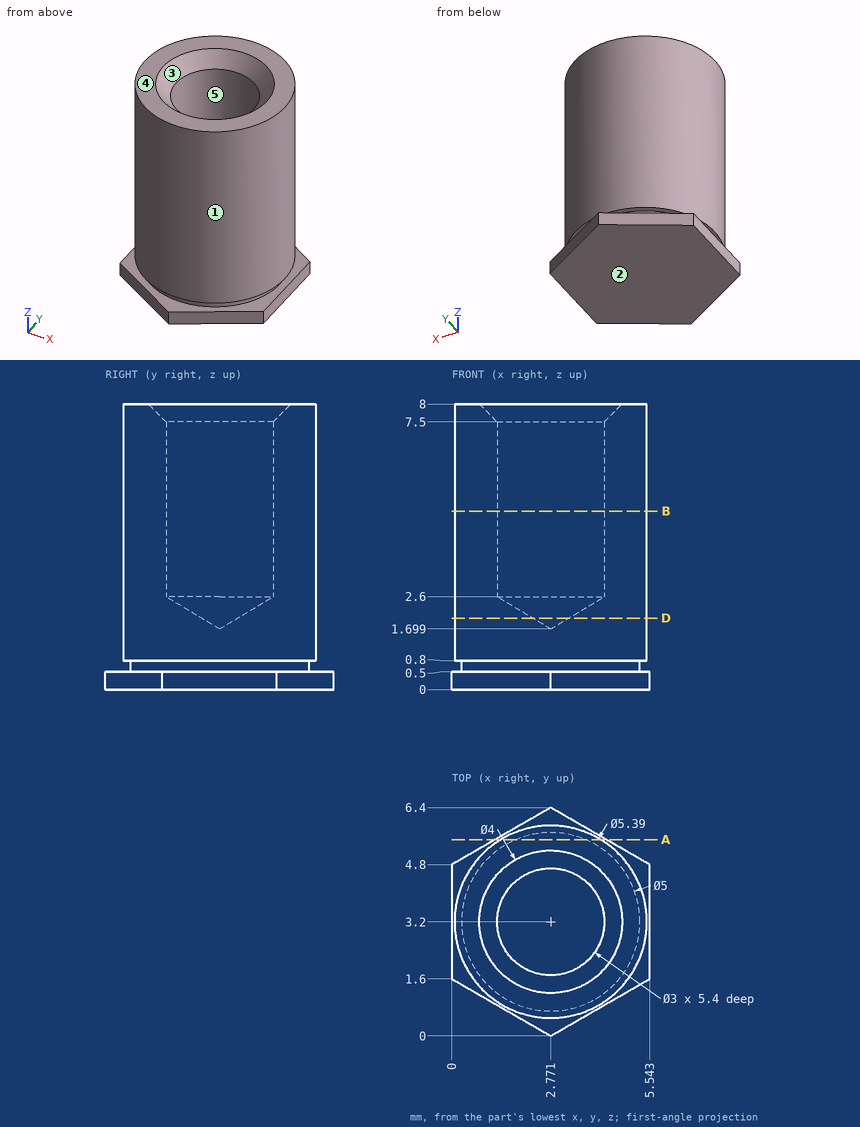
Verification items for this drawing (mm, ordinates from the low corner). A direction names the side the tool comes from. Give positions to 0.01 mm unless a question says otherwise; leave off trailing zeros. Loops run counter-clockwise (first coordinate to the right, second up) from the corner with the lowest first, then second, coordinate; pieces in that order, holes last. Notation, with made-up numbers: M -19,85 L -11,85 A19 cw -11,101 Z; hole C 66.25,33.25 d5. An arc over 180 degrees is marked long. Answer as a JSON object with one key per item and string values. Group by question number.
Q1. Cross-section at B-B on z = 5. Record the cut outline in (x, y) (1 decimal).
Q2. Release check for a two-part mould opening along X. For the marked faces 1, 2 and 3 record: released by +X, released by -X, zero draft, split by the parting line, or undercut.
Q3. Cross-section at A-A on y = 5.5. Record the cut outline in (x, z), then the cut area to 3 significant figures.
Q4. Go/stop test with flat-tipped pins: P1, Ø1.8, axis at x = 2.77, y = 3.2, coming from the +Z side; P2, Ø2, axis at x = 4, z = 5.5, coming from the +Y side (1 decimal). Record where each tip stops, or that it passes through.
Q5. Access from +Z, -Z, +X, -X, +Y, -Y to the whole of each face (thin tool, end or side, straight path). Record for the marked faces 4 and 5.
Q6. Material ranges on line 1 along Z through (x, y) = (0.6, 1.75); line 2 along X through (y, z) = (4.25, 7.25) (1 decimal); line 3 along Y through (x, z) = (2.5, 5.5) (1 decimal), recorded low to high. Write a range as [from, to].
Q7. Cross-section at D-D on z = 2. Record the cut outline in (x, y) (1 decimal), then the cut area to 3 significant figures.
Evaluation:
{
 "1": {"outline": "C 2.8,3.2 d5.4; hole C 2.8,3.2 d3"},
 "2": {"face 1": "split by the parting line", "face 2": "zero draft", "face 3": "undercut"},
 "3": {"outline": "M 1.21,0 L 4.33,0 L 4.33,0.5 L 3.75,0.5 L 3.75,0.8 L 4.18,0.8 L 4.18,8 L 1.37,8 L 1.37,0.8 L 1.79,0.8 L 1.79,0.5 L 1.21,0.5 Z", "area": "22.4 mm2"},
 "4": {"P1": "stops at z = 2.24", "P2": "stops at y = 5.9"},
 "5": {"face 4": "+Z, +X, -X, +Y, -Y", "face 5": "+Z"},
 "6": {"line 1": "z = [0, 0.5], [0.8, 8]", "line 2": "x = [0.3, 1.7], [3.8, 5.3]", "line 3": "y = [0.5, 1.7], [4.7, 5.9]"},
 "7": {"outline": "C 2.8,3.2 d5.4; hole C 2.8,3.2 d1", "area": "22.0 mm2"}
}
